Input: part model. Units: mm. Frame: model coordinates. A direction names the side the tool comes from. Coordinates: 2 decimals unless noted, no trailing zeros. Loops run counter-clockwise (first coordinate to the right, second up) from the corner with the lowest first, then second, coordinate; pieces in that order, holes last.
```python
from build123d import *

# Parameters (mm, degrees)
F0_W     = 56
F0_H     = 40
F0_W_2   = 40
F0_H_2   = 24
F1_DEPTH = 0.5
F0_W_3   = 58
F0_H_3   = 42
F2_DEPTH = 6.25
F3_W     = 5
F3_H     = 1.9
F4_DEPTH = 0.9
F5_R     = 0.8


# Not quite as in the source:
# - two fillets or chamfers of one size are made in one step
# - a pattern or mirror of a feature is missing from the dataset's text; its kind, count and spacing are read off the source's solid


with BuildPart() as f1:
    # F0 (on Top) → F1 (new body)
    with BuildSketch(Plane.XY):
        Rectangle(F0_W, F0_H)
        Rectangle(F0_W_2, F0_H_2, mode=Mode.SUBTRACT)
    extrude(amount=F1_DEPTH)

    # F0 (on Top) → F2 (join)
    with BuildSketch(Plane.XY):
        Rectangle(F0_W_3, F0_H_3)
        Rectangle(F0_W, F0_H, mode=Mode.SUBTRACT)
    extrude(amount=F2_DEPTH)

    # F3 (on face) → F4 (join)
    with BuildSketch(Plane(origin=(0, -20, 0), x_dir=(-1, 0, 0), z_dir=(0, 1, 0))):
        with Locations((0, 3.35)):
            Rectangle(F3_W, F3_H)
    f4 = extrude(amount=F4_DEPTH)

    # F4_copies: F4 across plane
    add(f4.mirror(Plane.ZX))

    # F5
    f5_edges = [f1.edges().sort_by_distance(p)[0] for p in [
        (0, -19.1, 4.3),
        (0, -19.1, 2.4),
        (29, 21, 3.125),
        (-29, 21, 3.125),
        (-29, -21, 3.125),
        (29, -21, 3.125),
        (0, 19.1, 4.3),
        (0, 19.1, 2.4),
    ]]
    fillet(f5_edges, radius=F5_R)


solid = f1.part
```
Item 1: Mould query, pull axis Y, two halves, no side actions, for faces 1 (the face through (29, 0, 3)), 2 (the face through (0, 21, 3)), 3 (the face through (0, 14, 0.5)), 4 (the face through (0, -21, 3)). Classes: +Y half, -Y half, draft (parallel to the pull), parting line (faces both ways), or undercut.
Result:
face 1: draft
face 2: +Y half
face 3: undercut
face 4: -Y half
Item 2: Section query D-D (x = -8). Output: boundary loops of the cut face in (y, z), then the cut area to 3 significant figures.
Result:
outline: (-21, 0) - (-12, 0) - (-12, 0.5) - (-20, 0.5) - (-20, 6.25) - (-21, 6.25) - close; (12, 0) - (21, 0) - (21, 6.25) - (20, 6.25) - (20, 0.5) - (12, 0.5) - close
area: 20.5 mm2
Item 3: Reachability of faces 5 (the face through (0, 14, 0)), 6 (the face through (28, 0, 3)) from +Z, -Z, +X, -X, +Y, -Y: full face, straight path, thin tool, end or side. Return the list, or none.
Result:
face 5: -Z, +X, -X, +Y, -Y
face 6: +Z
Item 4: Section query B-B (y = 8). Output: boundary loops of the cut face in (x, z).
Result:
outline: (-29, 0) - (-20, 0) - (-20, 0.5) - (-28, 0.5) - (-28, 6.25) - (-29, 6.25) - close; (20, 0) - (29, 0) - (29, 6.25) - (28, 6.25) - (28, 0.5) - (20, 0.5) - close
Item 5: Section query A-A (x = -1). Output: boundary loops of the cut face in (y, z).
Result:
outline: (-21, 0) - (-12, 0) - (-12, 0.5) - (-20, 0.5) - (-20, 2.4) - (-19.9, 2.4) arc R0.8 ccw to (-19.1, 3.2) - (-19.1, 3.5) arc R0.8 ccw to (-19.9, 4.3) - (-20, 4.3) - (-20, 6.25) - (-21, 6.25) - close; (12, 0) - (21, 0) - (21, 6.25) - (20, 6.25) - (20, 4.3) - (19.9, 4.3) arc R0.8 ccw to (19.1, 3.5) - (19.1, 3.2) arc R0.8 ccw to (19.9, 2.4) - (20, 2.4) - (20, 0.5) - (12, 0.5) - close
Item 6: Section query C-C (y = 14.5). Output: boundary loops of the cut face in (x, z), then the cut area to 3 significant figures.
Result:
outline: (-29, 0) - (29, 0) - (29, 6.25) - (28, 6.25) - (28, 0.5) - (-28, 0.5) - (-28, 6.25) - (-29, 6.25) - close
area: 40.5 mm2
Item 7: Line query: L1, parallel to X at y = 12, z = 1.25; L2, parallel to Y at x = -17, z = 6; L3, parallel to Z at x = -21.5, y = -4. Output: solid intervals per line, ascending.
Result:
L1: x = -29 to -28, 28 to 29
L2: y = -21 to -20, 20 to 21
L3: z = 0 to 0.5
Item 8: Contact query for a flat-ended pin moving along its axis: P1, Ø3, axis at x = 17, y = 4, coming from the +Z side. Output: stop coordinate, or through.
Result:
P1: passes through
